Build history of the part. All positions in model axes, mm. A direction names the side the tool comes from. Give positions to 0.01 mm unless a question says otherwise; leave off trailing zeros. Loops run counter-clockwise (first coordinate to the right, second up) from the corner with the lowest first, then second, coordinate; pieces in that order, holes last. Notation, with made-up numbers: M 14,35.25 L 62,35.25 A25 ccw 62,55.25 Z; hole C -1,19.5 d1. An arc over 180 degrees is marked long. Answer as a JSON object with one key per item and string values. Group by question number.
1. Slice it at A-A (z = -3.5). List the corners of the cut face in (x, y), then the cut area to 3 significant figures.
2. Drop flat-ended pins along their axis: pin 1 Ø1.5 at (x, z) = (32, -22.5) entering from +Y; pin 2 Ø1.5 at (y, z) = (3, -10.5) entering from -X; pin 3 Ø1.3 at (y, z) = (3, -21.5) entering from -X; pin 4 Ø2 at (x, y) = (37.5, 3) entering from -Z. Give the stop position or say it passes through.
3. Mould opens along Z. For faces 1 (the face through (47, 5, -22.424)), 2 (the face through (7, 5, -2.141)), 3 (the face through (50.8, 1, -19)) say: released by +Z, released by -Z, zero draft, split by the parting line, or undercut.
4. Slice it at D-D (z = -23). List the corners of the cut face in (x, y), then the cut area to 3 significant figures.
5. Slice it at B-B (x = 16.5). List the corners of the cut face in (y, z), then the cut area to 3 significant figures.
6. Slice it at C-C (y = 5.5). List the corners of the cut face in (x, z).
7. Drill centre lines: line 1 along X through (y, z) = (7, -5); line 2 along Z through (x, y) = (31, 4); line 3 along X through (y, z) = (8, -34.5). Where is each one in solid material? Low to high. Write a range as [from, to].
8. 3-axis set-ups, long thin cutter, end or side, ignore diameter. For faces 4 (the face through (49.19, 5, -19)), 5 (the face through (6.787, 5, -4)), 6 (the face through (29, 4.115, -23)), 7 (the face through (44.11, 5, -32)), 8 (the face through (29, 3, -26.859)): which of +Z, -Z, +X, -X, +Y, -Y reach the whole face in a straight line?
from build123d import *

# Parameters (mm, degrees)
SKETCH1_W           = 50.8
SKETCH1_H           = 38.1
BOSS_EXTRUDE1_DEPTH = 1.5748
SKETCH2_W           = 5.08
SKETCH2_H           = 7.62
BOSS_EXTRUDE2_DEPTH = 7.62
SKETCH3_R           = 3.127542457
SKETCH3_W           = 12.012072663
SKETCH3_H           = 7.683397829
BOSS_EXTRUDE3_DEPTH = 11.1252
SKETCH4_W           = 12.39083171
SKETCH4_H           = 7.62
BOSS_EXTRUDE4_DEPTH = 2.54
SKETCH5_W           = 6.49301225
SKETCH5_H           = 6.601229121
BOSS_EXTRUDE5_DEPTH = 1.27
SKETCH6_W           = 1.27
SKETCH6_H           = 4.49100014
BOSS_EXTRUDE6_DEPTH = 7.112
SKETCH7_R           = 1.645643818
SKETCH7_R_2         = 1.500472866
SKETCH7_R_3         = 1.42952807
SKETCH7_R_4         = 1.703993098
CUT_EXTRUDE1_DEPTH  = 7.112


with BuildPart() as part:
    # Sketch1 → Boss-Extrude1 (new body)
    with BuildSketch(Plane(origin=(0, 0, 0), x_dir=(1, 0, 0), z_dir=(0, 1, 0))):
        with Locations((25.4, 19.05)):
            Rectangle(SKETCH1_W, SKETCH1_H)
    extrude(amount=BOSS_EXTRUDE1_DEPTH)

    # Sketch2 → Boss-Extrude2 (add)
    with BuildSketch(Plane(origin=(0, 1.5748, 0), x_dir=(1, 0, 0), z_dir=(0, 1, 0))):
        with Locations((46.649948662, 6.474433462)):
            Rectangle(SKETCH2_W, SKETCH2_H)
        with Locations((46.649948662, 18.613569988)):
            Rectangle(SKETCH2_W, SKETCH2_H)
        with Locations((46.649948662, 31.703482685)):
            Rectangle(SKETCH2_W, SKETCH2_H)
    extrude(amount=BOSS_EXTRUDE2_DEPTH)

    # Sketch3 → Boss-Extrude3 (add)
    with BuildSketch(Plane(origin=(0, 1.5748, 0), x_dir=(1, 0, 0), z_dir=(0, 1, 0))):
        with Locations(Location((30.756735106, 33.361681168, 0), (0, 0, 90))):
            Circle(SKETCH3_R)
        with Locations((14.091336998, 32.658271508)):
            Rectangle(SKETCH3_W, SKETCH3_H)
    extrude(amount=BOSS_EXTRUDE3_DEPTH)

    # Sketch4 → Boss-Extrude4 (add)
    with BuildSketch(Plane(origin=(0, 1.5748, 0), x_dir=(1, 0, 0), z_dir=(0, 1, 0))):
        with Locations((28.727668778, 23.049379524)):
            Rectangle(SKETCH4_W, SKETCH4_H)
        with Locations((28.727668778, 10.22568033)):
            Rectangle(SKETCH4_W, SKETCH4_H)
    extrude(amount=BOSS_EXTRUDE4_DEPTH)

    # Sketch5 → Boss-Extrude5 (add)
    with BuildSketch(Plane(origin=(0, 1.5748, 0), x_dir=(1, 0, 0), z_dir=(0, 1, 0))):
        with Locations((10.087312777, 20.267439796)):
            Rectangle(SKETCH5_W, SKETCH5_H)
    extrude(amount=BOSS_EXTRUDE5_DEPTH)

    # Sketch6 → Boss-Extrude6 (add)
    with BuildSketch(Plane(origin=(0, 1.5748, 0), x_dir=(1, 0, 0), z_dir=(0, 1, 0))):
        with Locations((7.421698216, 4.386614002)):
            Rectangle(SKETCH6_W, SKETCH6_H)
        with Locations((10.559987471, 4.386614002)):
            Rectangle(SKETCH6_W, SKETCH6_H)
    extrude(amount=BOSS_EXTRUDE6_DEPTH)

    # Sketch7 → Cut-Extrude1 (cut)
    with BuildSketch(Plane(origin=(0, 1.5748, 0), x_dir=(1, 0, 0), z_dir=(0, 1, 0))):
        with Locations(Location((3.269649914, 3.169174205, 0), (0, 0, 270))):
            Circle(SKETCH7_R)
        with Locations(Location((38.98121729, 3.169174205, 0), (0, 0, 270))):
            Circle(SKETCH7_R_2)
        with Locations(Location((38.98121729, 34.660283618, 0), (0, 0, 270))):
            Circle(SKETCH7_R_3)
        with Locations(Location((3.269649914, 34.660283618, 0), (0, 0, 270))):
            Circle(SKETCH7_R_4)
    extrude(amount=-CUT_EXTRUDE1_DEPTH, mode=Mode.SUBTRACT)


solid = part.part
Established:
{
 "1": {"outline": "M 0,0 L 1.66,0 L 1.66,1.57 L 0,1.57 Z; M 4.88,0 L 37.52,0 L 37.52,1.57 L 11.19,1.57 L 11.19,8.69 L 9.92,8.69 L 9.92,1.57 L 8.06,1.57 L 8.06,8.69 L 6.79,8.69 L 6.79,1.57 L 4.88,1.57 Z; M 40.44,0 L 50.8,0 L 50.8,1.57 L 49.19,1.57 L 49.19,9.19 L 44.11,9.19 L 44.11,1.57 L 40.44,1.57 Z", "area": "127 mm^2"},
 "2": {"pin 1": "stops at y = 4.11", "pin 2": "stops at x = 22.53", "pin 3": "stops at x = 6.84", "pin 4": "passes through"},
 "3": {"face 1": "undercut", "face 2": "released by +Z", "face 3": "zero draft"},
 "4": {"outline": "M 0,0 L 50.8,0 L 50.8,1.57 L 34.92,1.57 L 34.92,4.11 L 22.53,4.11 L 22.53,1.57 L 13.33,1.57 L 13.33,2.84 L 6.84,2.84 L 6.84,1.57 L 0,1.57 Z", "area": "120 mm^2"},
 "5": {"outline": "M 0,-38.1 L 1.57,-38.1 L 1.57,-36.5 L 12.7,-36.5 L 12.7,-28.82 L 1.57,-28.82 L 1.57,0 L 0,0 Z", "area": "145 mm^2"},
 "6": {"outline": "M 6.79,-6.63 L 8.06,-6.63 L 8.06,-2.14 L 6.79,-2.14 Z; M 8.09,-36.5 L 20.1,-36.5 L 20.1,-28.82 L 8.09,-28.82 Z; M 9.92,-6.63 L 11.19,-6.63 L 11.19,-2.14 L 9.92,-2.14 Z; C 30.76,-33.36 d6.26; M 44.11,-35.51 L 49.19,-35.51 L 49.19,-27.89 L 44.11,-27.89 Z; M 44.11,-22.42 L 49.19,-22.42 L 49.19,-14.8 L 44.11,-14.8 Z; M 44.11,-10.28 L 49.19,-10.28 L 49.19,-2.66 L 44.11,-2.66 Z"},
 "7": {"line 1": "x = [6.79, 8.06], [9.92, 11.19], [44.11, 49.19]", "line 2": "z = [-36.48, -30.24], [-26.86, -19.24], [-14.04, -6.42]", "line 3": "x = [8.09, 20.1], [27.84, 33.67], [44.11, 49.19]"},
 "8": {"face 4": "+Z, -Z, +X, +Y", "face 5": "+Z, -Z, -X, +Y", "face 6": "+Z, -X, +Y", "face 7": "+Z, -Z, +Y", "face 8": "+X, -X, +Y"}
}
